Work out the finished part from the listing and answer in its coordinate system (mm). Face numbers are marked on the shaded views. Round coordinates to 2 decimals unless told otherwise and drop trailing zeros. Order: outer loops, then holes, each group sorted by start corner. A loop starts at its lowest first (then second) coordinate and runs counter-clockwise, first axis right, second up. Notation, with made-up numbers: (-19.5, 6) - (39.5, 6) arc R26 ccw to (39.5, 39) - close; hole circle Ø2 at (66, -30). An arc over 180 degrees is marked (long way). Use one line per item in the form item = value. Start each with the question number.
Q1. For a pull along Z with two mould halves and no side action, classify the marked faces 1, 2, 3 and 4 as +Z half, -Z half, draft (parallel to the pull), parting line (faces both ways), or undercut.
Q2. Given P1, Ø4, axis at y = 21.5, z = -59.5, coming from the +X side; P2, Ø10, axis at x = -63, z = -27, coming from the -Y side, each flat-ended and moving along its own axis, determine where each tip first touches the part or whether it passes through.
Q3. The part is cut by section A-A on z = -26. Determine the outline of the cut face in (x, y).
Q4. Find the intervals of material crossed by line 1 (Y direction, x = -50.5, z = -5); line 2 (Y direction, x = -99.5, z = -57.5); line 3 (Z direction, x = -102, y = -1), in increasing order. Write a range as [from, to].
Q5. The part is cut by section B-B on y = 17. Determine the outline of the cut face in (x, z).
Autodesk Inventor part; units mm, degrees
ref_plane "Work Plane1" through (-92, 0, -37.5) normal (0, 0, 1) x (1, 0, 0)
ref_plane "Work Plane2" through (-55, 0, -18) normal (1, 0, 0) x (0, 0, -1)
ref_plane "YZ Plane" through (0, 0, 0) normal (1, 0, 0) x (0, 1, 0)
sketch "Sketch1" plane through (0, 0, 0) normal (0, 1, 0) x (-1, 0, 0)
  line L0 (0, 0) -> (110, 0)
  line L1 (110, 0) -> (110, -75)
  line L2 (110, -75) -> (0, -75)
  line L3 (0, -75) -> (0, 0)
  dimension "d0" = 110
  dimension "d1" = 75
extrude "Extrusion1" add sketch "Sketch1" along normal blind 27.5
fillet "Fillet1" radius 18 4 edges at (-110, 13.75, 0) (0, 13.75, 0) (0, 13.75, -75) (-110, 13.75, -75)
sketch "Sketch2" plane through (0, 0, 0) normal (0, -1, 0) x (1, 0, 0)
  line L0 (-110.0023, 0) -> (-0.0023, 0) construction
  line L1 (-0.0023, 0) -> (-0.0023, -81.8008) construction
  line L2 (-0.0023, -81.8008) -> (-110.0023, -81.8008) construction
  line L3 (-110.0023, -81.8008) -> (-110.0023, 0) construction
  arc A0 (-92, 0) -> (-110, -18) centre (-92, -18) ccw
  line L4 (-110.0023, 0) -> (-92, -18)
  circle A1 centre (-98.8278, -11.1731) radius 6.8778
  point P0 (0, 0)
  dimension "d14" = 110
extrude "Extrusion2" add sketch "Sketch2" along normal blind 2
sketch "Sketch3" plane through (-98.8278, -2, -11.1731) normal (0, -1, 0) x (1, 0, 0)
  circle A0 centre (0, 0) radius 6.25
  point P0 (98.8278, 11.1731)
  dimension "d28" = 12.5
extrude "Extrusion3" add sketch "Sketch3" along normal blind 0.5
ref_plane "Work Plane1" through (-92, 0, -37.5) normal (0, 0, 1) x (1, 0, 0)
ref_plane "Work Plane2" through (-55, 0, -18) normal (1, 0, 0) x (0, 0, -1)
mirror "Mirror1" about plane through (-92, 0, -37.5) normal (0, 0, 1) of "Extrusion2", "Extrusion3"
mirror "Mirror2" about plane through (-55, 0, -18) normal (1, 0, 0) of "Extrusion2", "Extrusion3", "Mirror1"
fillet "Fillet2" radius 0.5 16 edges at (-5.2721, 27.5, -5.2721) (0, 27.5, -37.5) (-5.2721, 27.5, -69.7279) (-55, 27.5, -75) (-104.7279, 27.5, -69.7279) (-110, 27.5, -37.5) (-104.7279, 27.5, -5.2721) (-55, 27.5, 0) (-104.7279, 0, -5.2721) (-110, 0, -37.5) (-104.7279, 0, -69.7279) (-55, 0, -75) (-5.2721, 0, -69.7279) (0, 0, -37.5) (-5.2721, 0, -5.2721) (-55, 0, 0)
properties part number "OM5P-AC"
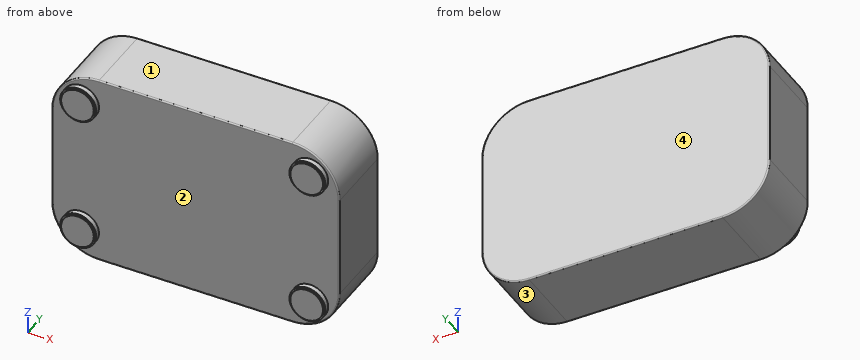
Found:
q1.face_1 = +Z half
q1.face_2 = undercut
q1.face_3 = -Z half
q1.face_4 = draft
q2.P1 = -0.01
q2.P2 = 0
q3.outline = (-110, 0.5) arc R0.5 ccw to (-109.5, 0) - (-0.5, 0) arc R0.5 ccw to (0, 0.5) - (0, 27) arc R0.5 ccw to (-0.5, 27.5) - (-109.5, 27.5) arc R0.5 ccw to (-110, 27) - close
q4.line_1 = [0, 27.5]
q4.line_2 = [-2, 27.5]
q4.line_3 = [-69.93, -57.72], [-17.28, -5.07]
q5.outline = (-110, -57) arc R18 ccw to (-92, -75) - (-18, -75) arc R18 ccw to (0, -57) - (0, -18) arc R18 ccw to (-18, 0) - (-92, 0) arc R18 ccw to (-110, -18) - close
